Here's how the part is built. I have some questions about the finished solid (model axes, mm). Face numbers are marked on the shaded views. Coordinates: 2 decimals unless noted, no trailing zeros. Loops run counter-clockwise (first coordinate to the right, second up) from the corner with the lowest first, then second, coordinate; pieces in that order, holes last. Notation, with made-up numbers: (-7.75, -34.75) - (44.25, -34.75) arc R10 cw to (44.25, -22.75) - close; hole circle Ø10 at (-36.75, 10.5). An arc over 180 degrees is marked (long way). Use a Markdown table: item, result.
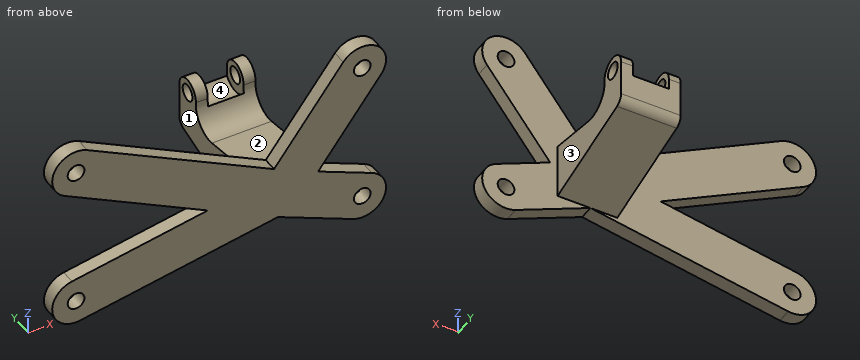
```python
from build123d import *

# Parameters (mm, degrees)
SKETCH1_R           = 1.75
BOSS_EXTRUDE1_DEPTH = 3
SKETCH2_R           = 1.75
BOSS_EXTRUDE2_DEPTH = 6.25
SKETCH3_R           = 3.75
CUT_EXTRUDE1_DEPTH  = 3.75


with BuildPart() as part:
    # Sketch1 → Boss-Extrude1 (new body)
    with BuildSketch(Plane(origin=(0, 0, 0), x_dir=(1, 0, 0), z_dir=(0, 1, 0))):
        with BuildLine():
            Line((-45.257003151, -18.071250027), (-15.343449858, -2.395547337))
            Line((-15.343449858, -2.395547337), (-43.796551891, 2.574578453))
            ThreePointArc((-43.796551891, 2.574578453), (-47.861611547, 8.360361891), (-42.075828109, 12.425421547))
            Line((-42.075828109, 12.425421547), (-0.628357098, 5.185467732))
            Line((-0.628357098, 5.185467732), (15.051932182, 12.077373444))
            ThreePointArc((15.051932182, 12.077373444), (21.641183444, 9.511877818), (19.075687818, 2.922626556))
            Line((19.075687818, 2.922626556), (7.812998809, -2.027625912))
            Line((7.812998809, -2.027625912), (21.047705857, -19.478647024))
            ThreePointArc((21.047705857, -19.478647024), (20.085162976, -26.483895857), (13.079914143, -25.521352976))
            Line((13.079914143, -25.521352976), (-1.427051817, -6.392756601))
            Line((-1.427051817, -6.392756601), (-40.615376849, -26.928749973))
            ThreePointArc((-40.615376849, -26.928749973), (-47.364939973, -24.820813151), (-45.257003151, -18.071250027))
        make_face()
        with Locations(Location((-42.93619, -22.5, 0), (0, 0, 270))):
            Circle(SKETCH1_R, mode=Mode.SUBTRACT)
        with Locations(Location((-42.93619, 7.5, 0), (0, 0, 270))):
            Circle(SKETCH1_R, mode=Mode.SUBTRACT)
        with Locations(Location((17.06381, 7.5, 0), (0, 0, 270))):
            Circle(SKETCH1_R, mode=Mode.SUBTRACT)
        with Locations(Location((17.06381, -22.5, 0), (0, 0, 270))):
            Circle(SKETCH1_R, mode=Mode.SUBTRACT)
    extrude(amount=BOSS_EXTRUDE1_DEPTH)

    # Sketch2 → Boss-Extrude2 (add, symmetric)
    with BuildSketch(Plane(origin=(0, 0, 0), x_dir=(0, 0, -1), z_dir=(1, 0, 0))):
        with BuildLine():
            Line((-6.392756601, 3), (-4.425253098, 14.158266845))
            ThreePointArc((-4.425253098, 14.158266845), (-5.653060678, 18.393683854), (-9.755984449, 20.0099404))
            ThreePointArc((-9.755984449, 20.0099404), (-12.99751387, 22.877891031), (-10, 26))
            Line((-10, 26), (-2.51201767, 26))
            ThreePointArc((-2.51201767, 26), (-1.294494812, 25.586706681), (-0.580166017, 24.51763809))
            Line((-0.580166017, 24.51763809), (5.185467732, 3))
            Line((5.185467732, 3), (-6.392756601, 3))
        make_face()
        with Locations((-10, 23)):
            Circle(SKETCH2_R, mode=Mode.SUBTRACT)
    extrude(amount=BOSS_EXTRUDE2_DEPTH, both=True)

    # Sketch3 → Cut-Extrude1 (cut, symmetric)
    with BuildSketch(Plane(origin=(0, 0, 0), x_dir=(0, 0, -1), z_dir=(1, 0, 0))):
        with Locations((-10, 23)):
            Circle(SKETCH3_R)
    extrude(amount=CUT_EXTRUDE1_DEPTH, both=True, mode=Mode.SUBTRACT)


solid = part.part
```
Q1. If we mould it in two halves opening along X, with no side actions, what happens to the marked faces 1, 2, 3 and 4? For each: pulls with the +X half, pulls with the -X half, needs draft (parallel to the pull), parting line crosses it, or undercut.
Check values:
| item | result |
|---|---|
| face 1 | pulls with the -X half |
| face 2 | needs draft |
| face 3 | pulls with the +X half |
| face 4 | undercut |
Q2. I want a section at A-A, the plane y = 23. Write out the boundary of the cut face in (x, z), then the cut area to 3 significant figures.
Check values:
| item | result |
|---|---|
| outline | (-6.25, 0.17) - (6.25, 0.17) - (6.25, 8.25) - (3.75, 8.25) - (3.75, 6.25) - (-3.75, 6.25) - (-3.75, 8.25) - (-6.25, 8.25) - close; (-6.25, 11.75) - (-3.75, 11.75) - (-3.75, 13) - (-6.25, 13) - close; (3.75, 11.75) - (6.25, 11.75) - (6.25, 13) - (3.75, 13) - close |
| area | 92.2 mm^2 |
Q3. Please list where these lines run through material, in increasing order: L1, parallel to Y at x = 5.3, z = 10; L2, parallel to Y at x = -9, z = 10; L3, parallel to X at y = 19.5, z = 2.5. Write a range as from..to.
Check values:
| item | result |
|---|---|
| L1 | 0..3, 20..21.25, 24.75..26 |
| L2 | 0..3 |
| L3 | -6.25..6.25 |
Q4. I want a section at C-C, the plane x = -18. Write out the boundary of the cut face in (y, z), then the cut area to 3 significant figures.
Check values:
| item | result |
|---|---|
| outline | (0, -8.22) - (3, -8.22) - (3, 1.93) - (0, 1.93) - close; (0, 3.79) - (3, 3.79) - (3, 15.08) - (0, 15.08) - close |
| area | 64.3 mm^2 |
Q5. I want a section at B-B, the plane z = -7.5. Write out the boundary of the cut face in (x, y).
Check values:
| item | result |
|---|---|
| outline | (-47.94, 0) - (-44.69, 0) - (-44.69, 3) - (-47.94, 3) - close; (-41.19, 0) - (-13.88, 0) - (-13.88, 3) - (-41.19, 3) - close; (4.64, 0) - (15.31, 0) - (15.31, 3) - (4.64, 3) - close; (18.81, 0) - (22.06, 0) - (22.06, 3) - (18.81, 3) - close |
Q6. Will these pins go through, and if not, where does the flat tip stop? P1, Ø14.5, axis at y = 18, z = 6, coming from the +X side; P2, Ø5, axis at y = 20.5, z = 0, coming from the -X side; P3, Ø3, axis at x = -37, y = 3.5, coming from the -Z side.
Check values:
| item | result |
|---|---|
| P1 | x = 6.25 |
| P2 | x = -6.25 |
| P3 | z = -11.79 |
Q7. I want a section at D-D, the plane z = 22.5. Write out the boundary of the cut face in (x, y).
Check values:
| item | result |
|---|---|
| outline | (-47.94, 0) - (-44.69, 0) - (-44.69, 3) - (-47.94, 3) - close; (-41.19, 0) - (-32.16, 0) - (-32.16, 3) - (-41.19, 3) - close; (10.79, 0) - (15.31, 0) - (15.31, 3) - (10.79, 3) - close; (18.81, 0) - (22.06, 0) - (22.06, 3) - (18.81, 3) - close |
